Check sheet for the drawn part. Datum: minimum x, y, z corner. Units: mm. Give positions to 0.01 mm unless a question says otherwise; leave off trailing zeros. Write each loop counter-clockwise with the first axis right and the second up, starting at its lowest first coordinate (ties: lowest second). Pieces come first, ordered by that corner, then holes. Notation, with made-up numbers: (15.25, 80) -> (65.25, 80) arc R16 cw to (65.25, 110) -> close; hole circle Ø5 at (4, 37.5). An arc over 180 degrees is marked (long way). Answer as CSV lines item,"result". Start each with the question number.
1) Sectioned sample at B-B on x = 10.6. Record the cut outline in (y, z), and give its area (3 significant figures).
2) Material ranges on L1, parallel to X at y = 0.95, z = 5; L2, parallel to Z at x = 10.5, y = 0.7; L3, parallel to X at y = 1.1, z = 3.75, recorded low to high.
3) Gauge pin test, flat end, axial feed: pin 1 Ø4 at (x, z) = (18, 4.5) entering from +Y. Record the tip position at first contact, or that the pin passes through.
4) Sectioned sample at C-C on z = 5.75. Record the cut outline in (x, y).
5) Sectioned sample at D-D on z = 1. Record the cut outline in (x, y).
6) Sectioned sample at A-A on y = 0.55. Record the cut outline in (x, z).
7) Mould release check, pull along X, two halves, no side actions. Record for the marked faces 1, 2, 3 and 4: released by +X, released by -X, zero draft, split by the parting line, or undercut.
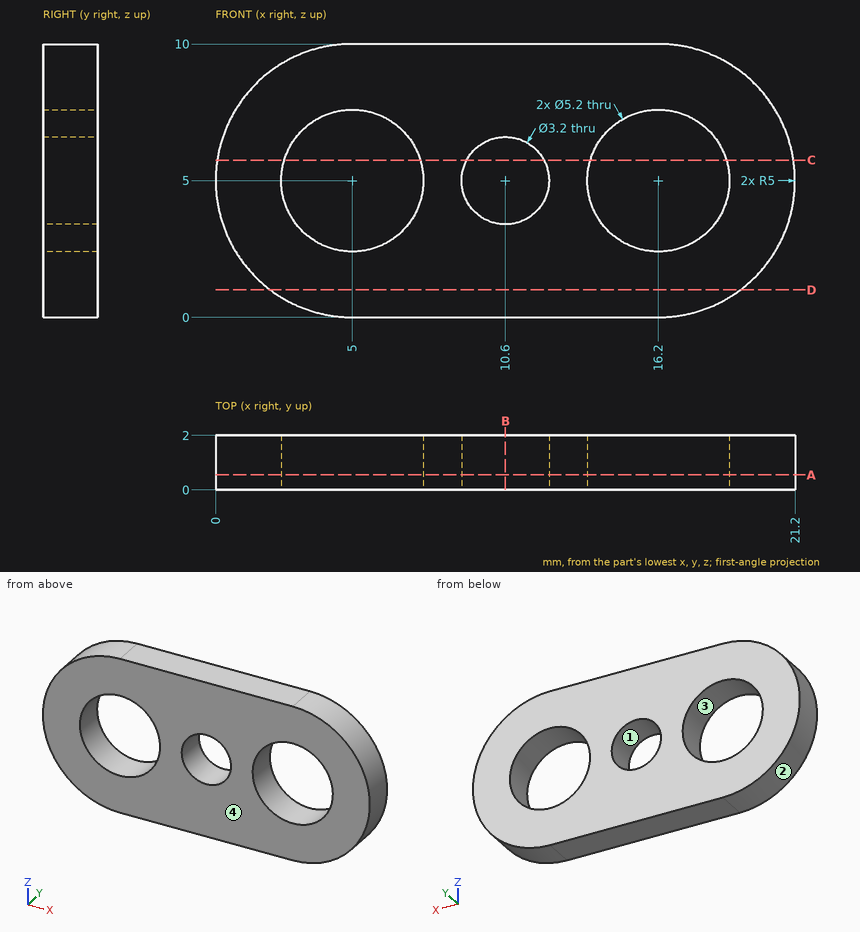
Ans:
1,outline,"(0, 0) -> (2, 0) -> (2, 3.4) -> (0, 3.4) -> close; (0, 6.6) -> (2, 6.6) -> (2, 10) -> (0, 10) -> close"
1,area,"13.6 mm²"
2,L1,"x = 0 to 2.4, 7.6 to 9, 12.2 to 13.6, 18.8 to 21.2"
2,L2,"z = 0 to 3.4, 6.6 to 10"
2,L3,"x = 0.16 to 2.72, 7.28 to 9.6, 11.6 to 13.92, 18.48 to 21.04"
3,pin 1,"stops at y = 2"
4,outline,"(0.06, 0) -> (2.51, 0) -> (2.51, 2) -> (0.06, 2) -> close; (7.49, 0) -> (9.19, 0) -> (9.19, 2) -> (7.49, 2) -> close; (12.01, 0) -> (13.71, 0) -> (13.71, 2) -> (12.01, 2) -> close; (18.69, 0) -> (21.14, 0) -> (21.14, 2) -> (18.69, 2) -> close"
5,outline,"(2, 0) -> (19.2, 0) -> (19.2, 2) -> (2, 2) -> close"
6,outline,"(5, 0) -> (16.2, 0) arc R5 ccw to (16.2, 10) -> (5, 10) arc R5 ccw to start; hole circle Ø5.2 at (5, 5); hole circle Ø3.2 at (10.6, 5); hole circle Ø5.2 at (16.2, 5)"
7,face 1,"undercut"
7,face 2,"released by -X"
7,face 3,"undercut"
7,face 4,"zero draft"
